Model file for the job. Use its own axes, mm. A direction names the side the tool comes from. Give positions to 0.01 mm unless a question says otherwise; leave off trailing zeros. Loops run counter-clockwise (first coordinate to the right, second up) from the corner with the lowest first, then second, coordinate; pieces in that order, holes last. Notation, with made-up numbers: (51, 2.5) - (105, 2.5) arc R26 ccw to (105, 19.5) - close; hole circle Ø4 at (42.25, 9.5). An arc over 180 degrees is marked (long way). Use a Markdown table: item, result.
from build123d import *

# Parameters (mm, degrees)
ESQUISSE1_W             = 100.4
ESQUISSE1_H             = 87
BOSS_EXTRU_1_DEPTH      = 50
ESQUISSE3_W             = 88.4
ESQUISSE3_H             = 75
ENL_V_MAT_EXTRU_1_DEPTH = 45
ESQUISSE5_W             = 3
ESQUISSE5_H             = 60
ENL_V_MAT_EXTRU_2_DEPTH = 45
ESQUISSE7_W             = 70
ESQUISSE7_H             = 3
ENL_V_MAT_EXTRU_3_DEPTH = 45
ESQUISSE8_W             = 100.4
ESQUISSE8_H             = 40
ENL_V_MAT_EXTRU_4_DEPTH = 45
ESQUISSE9_W             = 60
ESQUISSE9_H             = 87
ENL_V_MAT_EXTRU_5_DEPTH = 45


with BuildPart() as part:
    # Esquisse1 → Boss.-Extru.1 (new body)
    with BuildSketch(Plane.XY):
        Rectangle(ESQUISSE1_W, ESQUISSE1_H)
    extrude(amount=BOSS_EXTRU_1_DEPTH)

    # Esquisse3 → Enlèv. mat.-Extru.1 (cut)
    with BuildSketch(Plane.XY.offset(50)):
        Rectangle(ESQUISSE3_W, ESQUISSE3_H)
    extrude(amount=-ENL_V_MAT_EXTRU_1_DEPTH, mode=Mode.SUBTRACT)

    # Esquisse5 → Enlèv. mat.-Extru.2 (cut)
    with BuildSketch(Plane.XY.offset(50)):
        with Locations((-47.2, 0)):
            Rectangle(ESQUISSE5_W, ESQUISSE5_H)
    enl_v_mat_extru_2 = extrude(amount=-ENL_V_MAT_EXTRU_2_DEPTH, mode=Mode.SUBTRACT)

    # Symétrie1: Enlèv. mat.-Extru.2 across plane
    add(enl_v_mat_extru_2.mirror(Plane(origin=(0, 0, 0), x_dir=(0, 0, 1), z_dir=(1, 0, 0))), mode=Mode.SUBTRACT)

    # Esquisse7 → Enlèv. mat.-Extru.3 (cut)
    with BuildSketch(Plane.XY.offset(50)):
        with Locations((0, 40.5)):
            Rectangle(ESQUISSE7_W, ESQUISSE7_H)
    enl_v_mat_extru_3 = extrude(amount=-ENL_V_MAT_EXTRU_3_DEPTH, mode=Mode.SUBTRACT)

    # Symétrie2: Enlèv. mat.-Extru.3 across plane
    add(enl_v_mat_extru_3.mirror(Plane.ZX), mode=Mode.SUBTRACT)

    # Esquisse8 → Enlèv. mat.-Extru.4 (cut)
    with BuildSketch(Plane.XY.offset(50)):
        Rectangle(ESQUISSE8_W, ESQUISSE8_H)
    extrude(amount=-ENL_V_MAT_EXTRU_4_DEPTH, mode=Mode.SUBTRACT)

    # Esquisse9 → Enlèv. mat.-Extru.5 (cut)
    with BuildSketch(Plane.XY.offset(50)):
        Rectangle(ESQUISSE9_W, ESQUISSE9_H)
    extrude(amount=-ENL_V_MAT_EXTRU_5_DEPTH, mode=Mode.SUBTRACT)


solid = part.part
(1) Mould opens along Y. For faces 3 (the flat face through (-1, -43.5, 2)), 4 (the flat face through (44.4, -34.2, 50)), 5 (the flat face through (-47, 30, 28)) say: pulls with the +Y half, pulls with the -Y half, needs draft (parallel to the pull), parting line crosses it, or undercut.
Computed:
| item | result |
|---|---|
| face 3 | pulls with the -Y half |
| face 4 | needs draft |
| face 5 | undercut |
(2) 3-axis set-ups, long thin cutter, end or side, ignore diameter. For faces 1 (the flat face through (44.4, 34.5, 50)), 2 (the flat face through (-35, -40, 28)): which of +Z, -Z, +X, -X, +Y, -Y reach the whole face in a straight line?
Computed:
| item | result |
|---|---|
| face 1 | +Z, +X, -X, +Y, -Y |
| face 2 | +Z |
(3) Slice it at B-B, the plane x = 42. Write the cut outline in (y, z), plus the area to 3 significant figures.
Computed:
| item | result |
|---|---|
| outline | (-43.5, 0) - (43.5, 0) - (43.5, 50) - (37.5, 50) - (37.5, 5) - (-37.5, 5) - (-37.5, 50) - (-43.5, 50) - close |
| area | 975 mm² |
(4) Slice it at D-D, the plane y = -33. Write the cut outline in (x, z).
Computed:
| item | result |
|---|---|
| outline | (-50.2, 0) - (50.2, 0) - (50.2, 50) - (44.2, 50) - (44.2, 5) - (-44.2, 5) - (-44.2, 50) - (-50.2, 50) - close |
(5) Slice it at C-C, the plane z = 37. Count the separate pieces of the cut face and the enclosed holes in it, plus the area to 3 significant figures.
Computed:
| item | result |
|---|---|
| separate pieces | 4 |
| enclosed holes | 0 |
| area | 725 mm² |
(6) Slice it at A-A, the plane y = -21.5. Write the cut outline in (x, z), plus the area to 3 significant figures.
Computed:
| item | result |
|---|---|
| outline | (-50.2, 0) - (50.2, 0) - (50.2, 50) - (48.7, 50) - (48.7, 5) - (45.7, 5) - (45.7, 50) - (44.2, 50) - (44.2, 5) - (-44.2, 5) - (-44.2, 50) - (-45.7, 50) - (-45.7, 5) - (-48.7, 5) - (-48.7, 50) - (-50.2, 50) - close |
| area | 772 mm² |
(7) Pin check, flat tips, straight feed: P1, Ø2, axis at x = -10.5, y = -0.5, coming from the +Z side; P2, Ø12, axis at x = -21, z = 32, coming from the -Y side. Stop position of each tip, or through.
Computed:
| item | result |
|---|---|
| P1 | z = 5 |
| P2 | through |
(8) Drill centre lines: probe 1 along Y at (x, z) = (-31, 22); probe 2 along X at (y, z) = (-21, 14); probe 3 along X at (y, z) = (-34, 9). Where is each one in solid material? Low to high. Write a range as [from, to].
Computed:
| item | result |
|---|---|
| probe 1 | [-43.5, -42], [-39, -37.5], [37.5, 39], [42, 43.5] |
| probe 2 | [-50.2, -48.7], [-45.7, -44.2], [44.2, 45.7], [48.7, 50.2] |
| probe 3 | [-50.2, -44.2], [44.2, 50.2] |
